The listing builds one solid part. Answer for the finished solid, in the listing's coordinates (mm). A direction names the side the tool comes from. Give positions to 0.01 mm unless a question says otherwise; leave off trailing zeros. Write each loop counter-clockwise with the first axis right and the second up, starting at its lowest first coordinate (ties: lowest second). Pieces come first, ordered by that corner, then holes. Notation, with made-up numbers: M -21.75,20.5 L -4.75,20.5 A32 ccw -4.75,51.5 Z; hole C 49.5,58 d3. An arc over 180 degrees is marked long. Return JSON: item names as keys, results as strings.
from build123d import *

# Parameters (mm, degrees)
SKETCH_1_R          = 1.15
EXTRUDE_1_DEPTH     = 4
SKETCH_2_R          = 1
CUT_EXTRUDE_1_DEPTH = 3.5


with BuildPart() as part:
    # 草图1 → 凸台-拉伸1 (new body)
    with BuildSketch(Plane.XY):
        with BuildLine():
            Line((2, 0), (2, -5))
            Line((2, -5), (-2, -5))
            Line((-2, -5), (-2, 0))
            ThreePointArc((-2, 0), (0, 2), (2, 0))
        make_face()
        Circle(SKETCH_1_R, mode=Mode.SUBTRACT)
    extrude(amount=EXTRUDE_1_DEPTH)

    # 草图2 → 切除-拉伸1 (cut)
    with BuildSketch(Plane.XZ.offset(5)):
        with Locations(Location((0, 2, 0), (0, 0, 270))):
            Circle(SKETCH_2_R)
    extrude(amount=-CUT_EXTRUDE_1_DEPTH, mode=Mode.SUBTRACT)


solid = part.part
Item 1: A cutting plane is placed at A-A, the plane x = 0. Write down the section's boundary in (y, z), plus the area to 3 significant figures.
Geometry results:
{"outline": "M -5,0 L -1.15,0 L -1.15,4 L -5,4 L -5,3 L -1.5,3 L -1.5,1 L -5,1 Z; M 1.15,0 L 2,0 L 2,4 L 1.15,4 Z", "area": "11.8 mm2"}
Item 2: A cutting plane is placed at B-B, the plane z = 2. Write down the section's boundary in (x, y).
Geometry results:
{"outline": "M -2,-5 L -1,-5 L -1,-1.5 L 1,-1.5 L 1,-5 L 2,-5 L 2,0 A2 ccw -2,0 Z; hole C 0,0 d2.3"}
Item 3: Determine the mould class of faces 3 (the flat face through (0, -1.5, 2)), 4 (the cylindrical face through (-0.91, -0.7, 1.97)), 5 (the flat face through (0, -2, 0)), 6 (the flat face through (-2, -3, 2)) for opening direction X: +X half, -X half, draft (parallel to the pull), parting line (faces both ways), or undercut.
Geometry results:
{"face 3": "undercut", "face 4": "undercut", "face 5": "draft", "face 6": "-X half"}
Item 4: Given pin 1 Ø1 at (x, y) = (-1.5, 0) entering from -Z; pin 2 Ø1.2 at (x, z) = (0, 2) entering from -Y, each flat-ended and moving along its own axis, determine where each tip first touches the part or whether it passes through.
Geometry results:
{"pin 1": "stops at z = 0", "pin 2": "stops at y = -1.5"}
Item 5: A cutting plane is placed at D-D, the plane y = -2.25. Write down the section's boundary in (x, z).
Geometry results:
{"outline": "M -2,0 L 2,0 L 2,4 L -2,4 Z; hole C 0,2 d2"}
Item 6: Find the intervals of material crossed by line 1 (Y direction, x = 0, z = 2.2); line 2 (Z direction, x = 0.25, y = -3.5); line 3 (Y direction, x = 0.7, z = 2.3), in increasing order.
Geometry results:
{"line 1": "y = -1.5 to -1.15, 1.15 to 2", "line 2": "z = 0 to 1.03, 2.97 to 4", "line 3": "y = -1.5 to -0.91, 0.91 to 1.87"}
Item 7: A cutting plane is placed at C-C, the plane y = 0.75. Write down the section's boundary in (x, z).
Geometry results:
{"outline": "M -1.85,0 L -0.87,0 L -0.87,4 L -1.85,4 Z; M 0.87,0 L 1.85,0 L 1.85,4 L 0.87,4 Z"}
Item 8: Which of the six approach directions +Z, -Z, +X, -X, +Y, -Y give full straight-line access (tool end or side, diameter ignored) to faces 1 (the cylindrical face through (-0.6, -3.3, 2.8)), 2 (the cylindrical face through (0, 2, 2))?
Geometry results:
{"face 1": "-Y", "face 2": "+Z, -Z, +Y"}
